from build123d import *

# Parameters (mm, degrees)
F1_DEPTH = 1200
F2_R     = 2


# Not quite as in the source:
# - a feature names something its author has since deleted; it is built from what else it names


with BuildPart() as f1:
    # F0 (on Right) → F1 (new body)
    with BuildSketch(Plane.YZ):
        Polygon((-18.8378913403, 177.8021101952), (-18.8378913403, 154.8021101952), (-16.8378913403, 154.8021101952), (-16.8378913403, 179.8021101952), (-56.8378913403, 179.8021101952), (-56.8378913403, 79.8021101952), (-29.8378913403, 79.8021101952), (-29.8378913403, 53.8021101952), (-27.8378913403, 53.8021101952), (-27.8378913403, 81.8021101952), (-54.8378913403, 81.8021101952), (-54.8378913403, 177.8021101952), align=None)
    extrude(amount=F1_DEPTH)

    # F2
    f2_edges = [f1.edges().sort_by_distance(p)[0] for p in [
        (600, -56.837891, 179.80211),
        (600, -16.837891, 179.80211),
        (600, -56.837891, 79.80211),
        (600, -27.837891, 81.80211),
        (600, -54.837891, 81.80211),
        (600, -29.837891, 79.80211),
        (600, -18.837891, 177.80211),
        (600, -54.837891, 177.80211),
    ]]
    fillet(f2_edges, radius=F2_R)


solid = f1.part
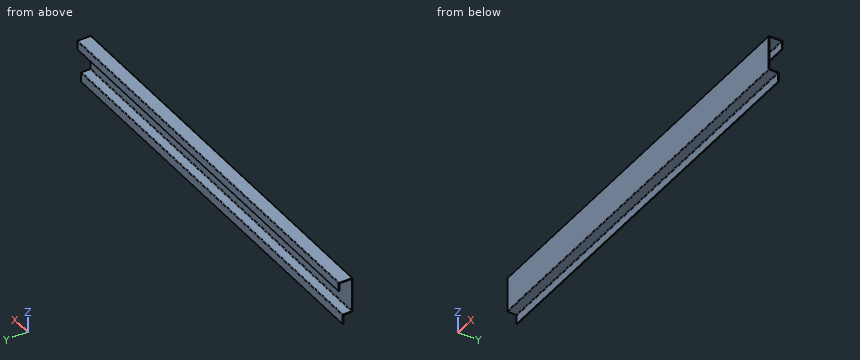
Geometry: final body of the model. Coordinates: model frame, mm. Give positions to 0.01 mm unless a question says otherwise; leave off trailing zeros. Loops run counter-clockwise (first coordinate to the right, second up) from the corner with the lowest first, then second, coordinate; pieces in that order, holes last. Notation, with made-up numbers: (60, -6.75) -> (99, -6.75) arc R26 ccw to (99, 14.25) -> close; hole circle Ø9 at (-11.5, -24). An arc over 180 degrees is marked (long way). Put each result on its own line as item: value.
1. Cut plane B-B (x = 421.5). Return the cut outline in (y, z).
Taken from the geometry:
outline: (-56.84, 81.8) arc R2 ccw to (-54.84, 79.8) -> (-31.84, 79.8) arc R2 cw to (-29.84, 77.8) -> (-29.84, 53.8) -> (-27.84, 53.8) -> (-27.84, 79.8) arc R2 ccw to (-29.84, 81.8) -> (-52.84, 81.8) arc R2 cw to (-54.84, 83.8) -> (-54.84, 175.8) arc R2 cw to (-52.84, 177.8) -> (-20.84, 177.8) arc R2 cw to (-18.84, 175.8) -> (-18.84, 154.8) -> (-16.84, 154.8) -> (-16.84, 177.8) arc R2 ccw to (-18.84, 179.8) -> (-54.84, 179.8) arc R2 ccw to (-56.84, 177.8) -> close
2. Ray query, line 1 along Z through (x, y) = (1080.5, -31); line 2 along Z through (x, y) = (714, -49.5); line 3 along Y through (x, z) = (171, 158.5). Return the intervals inside material, ascending. Write a range as [from, to].
Taken from the geometry:
line 1: z = [79.62, 81.8], [177.8, 179.8]
line 2: z = [79.8, 81.8], [177.8, 179.8]
line 3: y = [-56.84, -54.84], [-18.84, -16.84]
3. Pin query (flat end, axial travel): P1, Ø7, axis at x = 471.5, y = -45.5, coming from the -Z side; P2, Ø13, axis at x = 402, z = 71.5, coming from the +Y side; P3, Ø7, axis at x = 643, z = 68, coming from the -Y side. Return the tip coordinate at first contact, or that it passes through.
Taken from the geometry:
P1: stops at z = 79.8
P2: stops at y = -27.84
P3: stops at y = -29.84
4. Cut plane C-C (z = 67). Return the cut outline in (x, y).
Taken from the geometry:
outline: (0, -29.84) -> (1200, -29.84) -> (1200, -27.84) -> (0, -27.84) -> close
5. Cut plane A-A (y = -46). Return the cut outline in (x, z), plus the area to 3 significant figures.
Taken from the geometry:
outline: (0, 79.8) -> (1200, 79.8) -> (1200, 81.8) -> (0, 81.8) -> close; (0, 177.8) -> (1200, 177.8) -> (1200, 179.8) -> (0, 179.8) -> close
area: 4,800 mm2
